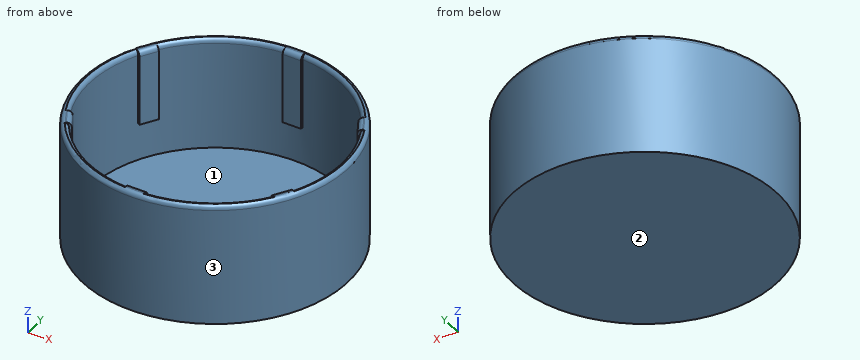
from build123d import *

# Parameters (mm, degrees)
F0_R         = 7.1
F1_DEPTH     = 0.5
F2_R         = 7.1
F2_R_2       = 6.7
F3_DEPTH     = 6
F4_W         = 1
F4_H         = 0.3
F5_DEPTH     = 4
F6_R         = 0.25
F7_T4_ANGLE  = 62.1313472273
F7_T10_ANGLE = 62.1313472273
F7_T16_ANGLE = 62.1313472273
F7_T22_ANGLE = 62.1313472273
F7_T28_ANGLE = 31.0651476548
F7_T33_ANGLE = 62.1313472273
F7_T39_ANGLE = 31.0651476548
F8_R         = 0.25


# Not quite as in the source:
# - a fillet or chamfer that OpenCascade refuses, or shapes differently, is made with other operations: its cross-section is extruded or revolved along the edge and cut away or added


with BuildPart() as f1:
    # F0 (on Top) → F1 (new body)
    with BuildSketch(Plane.XY):
        Circle(F0_R)
    extrude(amount=F1_DEPTH)

    # F2 (on face) → F3 (join)
    with BuildSketch(Plane.XY.offset(0.5)):
        Circle(F2_R)
        Circle(F2_R_2, mode=Mode.SUBTRACT)
    extrude(amount=F3_DEPTH)

    # F4 (on face) → F5 (join)
    with BuildSketch(Plane.XY.offset(6.5)):
        with Locations((0, 6.7)):
            Rectangle(F4_W, F4_H)
        Polygon((-5.9224663948, 2.8419872981), (-5.4224663948, 3.7080127019), (-5.6822740159, 3.8580127019), (-6.1822740159, 2.9919872981), align=None)
        Polygon((-5.4224663948, -3.7080127019), (-5.9224663948, -2.8419872981), (-6.1822740159, -2.9919872981), (-5.6822740159, -3.8580127019), align=None)
        with Locations((0, -6.7)):
            Rectangle(F4_W, F4_H)
        Polygon((5.9224663948, -2.8419872981), (5.4224663948, -3.7080127019), (5.6822740159, -3.8580127019), (6.1822740159, -2.9919872981), align=None)
        Polygon((5.4224663948, 3.7080127019), (5.9224663948, 2.8419872981), (6.1822740159, 2.9919872981), (5.6822740159, 3.8580127019), align=None)
    extrude(amount=-F5_DEPTH)

    # F6
    f6_edges = [f1.edges().sort_by_distance(p)[0] for p in [
        (-7.1, 0, 6.5),
    ]]
    fillet(f6_edges, radius=F6_R)

    # F7: fillet of radius 0.25 on 6 edges, made by hand


with BuildPart() as f7_tool2:
    # F7_s3 → F7_t4 (revolve)
    with BuildSketch(Plane(origin=(0, 0, 0), x_dir=(0, 0, 1), z_dir=(-0.4838067947, 0.8751748313, 0))):
        with BuildLine():
            ThreePointArc((6.5, -6.95), (6.4267766953, -6.7732233047), (6.25, -6.7))
            Line((6.25, -6.7), (6.5, -6.7))
            Line((6.5, -6.7), (6.5, -6.95))
        make_face()
    revolve(axis=Axis((0, 0, 6.5), (0, 0, 1)), revolution_arc=F7_T4_ANGLE)

    split(bisect_by=Plane.YZ.offset(-0.5), keep=Keep.BOTTOM)

    split(bisect_by=Plane(origin=(0.25, -0.4330127019, 0), x_dir=(0, 0, 1), z_dir=(0.5, -0.8660254038, 0)), keep=Keep.TOP)


with BuildPart() as f1_1:
    add(f1.part)

    # F7_t1: cut F7_tool2
    add(f7_tool2.part, mode=Mode.SUBTRACT)


with BuildPart() as f7_tool8:
    # F7_s9 → F7_t10 (revolve)
    with BuildSketch(Plane(origin=(0, 0, 0), x_dir=(0, 0, 1), z_dir=(0.5160202393, 0.8565763904, 0))):
        with BuildLine():
            ThreePointArc((6.5, -6.95), (6.4267766953, -6.7732233047), (6.25, -6.7))
            Line((6.25, -6.7), (6.5, -6.7))
            Line((6.5, -6.7), (6.5, -6.95))
        make_face()
    revolve(axis=Axis((0, 0, 6.5), (0, 0, 1)), revolution_arc=F7_T10_ANGLE)

    split(bisect_by=Plane(origin=(-0.25, 0.4330127019, 0), x_dir=(0, 0, 1), z_dir=(-0.5, 0.8660254038, 0)), keep=Keep.TOP)

    split(bisect_by=Plane(origin=(-0.25, -0.4330127019, 0), x_dir=(0, 0, 1), z_dir=(-0.5, -0.8660254038, 0)), keep=Keep.TOP)


with BuildPart() as f1_2:
    add(f1_1.part)

    # F7_t7: cut F7_tool8
    add(f7_tool8.part, mode=Mode.SUBTRACT)


with BuildPart() as f7_tool14:
    # F7_s15 → F7_t16 (revolve)
    with BuildSketch(Plane(origin=(0, 0, 0), x_dir=(0, 0, 1), z_dir=(0.999827034, -0.0185984409, 0))):
        with BuildLine():
            ThreePointArc((6.5, -6.95), (6.4267766953, -6.7732233047), (6.25, -6.7))
            Line((6.25, -6.7), (6.5, -6.7))
            Line((6.5, -6.7), (6.5, -6.95))
        make_face()
    revolve(axis=Axis((0, 0, 6.5), (0, 0, 1)), revolution_arc=F7_T16_ANGLE)

    split(bisect_by=Plane(origin=(0.25, 0.4330127019, 0), x_dir=(0, 0, 1), z_dir=(0.5, 0.8660254038, 0)), keep=Keep.TOP)

    split(bisect_by=Plane.YZ.offset(-0.5), keep=Keep.BOTTOM)


with BuildPart() as f1_3:
    add(f1_2.part)

    # F7_t13: cut F7_tool14
    add(f7_tool14.part, mode=Mode.SUBTRACT)


with BuildPart() as f7_tool20:
    # F7_s21 → F7_t22 (revolve)
    with BuildSketch(Plane(origin=(0, 0, 0), x_dir=(0, 0, 1), z_dir=(0.4838067947, -0.8751748313, 0))):
        with BuildLine():
            ThreePointArc((6.5, -6.95), (6.4267766953, -6.7732233047), (6.25, -6.7))
            Line((6.25, -6.7), (6.5, -6.7))
            Line((6.5, -6.7), (6.5, -6.95))
        make_face()
    revolve(axis=Axis((0, 0, 6.5), (0, 0, 1)), revolution_arc=F7_T22_ANGLE)

    split(bisect_by=Plane.YZ.offset(0.5), keep=Keep.TOP)

    split(bisect_by=Plane(origin=(-0.25, 0.4330127019, 0), x_dir=(0, 0, 1), z_dir=(-0.5, 0.8660254038, 0)), keep=Keep.TOP)


with BuildPart() as f1_4:
    add(f1_3.part)

    # F7_t19: cut F7_tool20
    add(f7_tool20.part, mode=Mode.SUBTRACT)


with BuildPart() as f7_tool26:
    # F7_s27 → F7_t28 (revolve)
    with BuildSketch(Plane(origin=(0, 0, 0), x_dir=(0, 0, 1), z_dir=(-0.5160123762, -0.8565811273, 0))):
        with BuildLine():
            ThreePointArc((6.5, -6.95), (6.4267766953, -6.7732233047), (6.25, -6.7))
            Line((6.25, -6.7), (6.5, -6.7))
            Line((6.5, -6.7), (6.5, -6.95))
        make_face()
    revolve(axis=Axis((0, 0, 6.5), (0, 0, 1)), revolution_arc=F7_T28_ANGLE)

    split(bisect_by=Plane(origin=(0.25, 0.4330127019, 0), x_dir=(0, 0, 1), z_dir=(0.5, 0.8660254038, 0)), keep=Keep.TOP)


with BuildPart() as f1_5:
    add(f1_4.part)

    # F7_t25: cut F7_tool26
    add(f7_tool26.part, mode=Mode.SUBTRACT)


with BuildPart() as f7_tool31:
    # F7_s32 → F7_t33 (revolve)
    with BuildSketch(Plane(origin=(0, 0, 0), x_dir=(0, 0, 1), z_dir=(-0.999827034, 0.0185984409, 0))):
        with BuildLine():
            ThreePointArc((6.5, -6.95), (6.4267766953, -6.7732233047), (6.25, -6.7))
            Line((6.25, -6.7), (6.5, -6.7))
            Line((6.5, -6.7), (6.5, -6.95))
        make_face()
    revolve(axis=Axis((0, 0, 6.5), (0, 0, 1)), revolution_arc=F7_T33_ANGLE)

    split(bisect_by=Plane(origin=(-0.25, -0.4330127019, 0), x_dir=(0, 0, 1), z_dir=(-0.5, -0.8660254038, 0)), keep=Keep.TOP)

    split(bisect_by=Plane.YZ.offset(0.5), keep=Keep.TOP)


with BuildPart() as f1_6:
    add(f1_5.part)

    # F7_t30: cut F7_tool31
    add(f7_tool31.part, mode=Mode.SUBTRACT)


with BuildPart() as f7_tool37:
    # F7_s38 → F7_t39 (revolve)
    with BuildSketch(Plane.XZ):
        with BuildLine():
            ThreePointArc((6.95, 6.5), (6.7732233047, 6.4267766953), (6.7, 6.25))
            Line((6.7, 6.25), (6.7, 6.5))
            Line((6.7, 6.5), (6.95, 6.5))
        make_face()
    revolve(axis=Axis((0, 0, 6.5), (0, 0, 1)), revolution_arc=F7_T39_ANGLE)

    split(bisect_by=Plane(origin=(0.25, -0.4330127019, 0), x_dir=(0, 0, 1), z_dir=(0.5, -0.8660254038, 0)), keep=Keep.TOP)


with BuildPart() as f1_7:
    add(f1_6.part)

    # F7_t36: cut F7_tool37
    add(f7_tool37.part, mode=Mode.SUBTRACT)

    # F8
    f8_edges = [f1_7.edges().sort_by_distance(p)[0] for p in [
        (-5.672466, 3.275, 6.5),
        (0, 6.55, 6.5),
        (5.672466, 3.275, 6.5),
        (5.672466, -3.275, 6.5),
        (0, -6.55, 6.5),
        (-5.672466, -3.275, 6.5),
    ]]
    fillet(f8_edges, radius=F8_R)


solid = f1_7.part
The listing builds one solid part. Answer for the finished solid, in the listing's coordinates (mm). Face numbers are marked on the shaded views. Give positions to 0.01 mm unless a question says otherwise; leave off trailing zeros. Write each loop counter-clockwise with the first axis right and the second up, starting at its lowest first coordinate (ties: lowest second). Pieces come first, ordered by that corner, then holes.
Item 1: Section A-A, the plane x = 0 is taken. Write down the section's boundary in (y, z), plus the area to 3 significant figures.
Item 2: Find the intervals of material crossed by line 1 along Y through (x, z) = (0, 5.05); line 2 along Y through (x, z) = (0, 1.95); line 3 along X through (y, z) = (-6, 5), in increasing order.
Item 3: Flat-ended cylindrical pins translate along their axes: P1, Ø0.5, axis at x = 5.5, y = 3.5, coming from the -Z side; P2, Ø2, axis at y = 2.5, z = 5.5, coming from the +X side; P3, Ø1, axis at x = 2.5, z = 3, coming from the -Y side; P4, Ø3, axis at y = 5, z = 5, coming from the +X side. Find the tip coordinate at first contact, or state that the pin passes through.
Item 4: Determine the mould class of the marked faces 1, 2 and 3 for opening direction Y: released by +Y, released by -Y, zero draft, split by the parting line, or undercut.
Item 5: Section B-B, the plane z = 5.75 is taken. Write down the section's boundary in (x, y).
Item 6: Section C-C, the plane z = 1.75 is taken. Write down the section's boundary in (x, y), plus the area to 3 significant figures.
Completed:
1. outline: (-7.1, 0) - (7.1, 0) - (7.1, 6.25) arc R0.25 ccw to (6.85, 6.5) - (6.8, 6.5) arc R0.25 ccw to (6.55, 6.25) - (6.55, 2.5) - (6.7, 2.5) - (6.7, 0.5) - (-6.7, 0.5) - (-6.7, 2.5) - (-6.55, 2.5) - (-6.55, 6.25) arc R0.25 ccw to (-6.8, 6.5) - (-6.85, 6.5) arc R0.25 ccw to (-7.1, 6.25) - close
1. area: 13.0 mm2
2. line 1: y = -7.1 to -6.55, 6.55 to 7.1
2. line 2: y = -7.1 to -6.7, 6.7 to 7.1
2. line 3: x = -3.8 to -2.98, 2.98 to 3.8
3. P1: stops at z = 0
3. P2: stops at x = 6.94
3. P3: stops at y = -6.81
3. P4: stops at x = 6.18
4. face 1: undercut
4. face 2: zero draft
4. face 3: split by the parting line
5. outline: circle Ø14.2 at (0, 0); hole (-6.04, -2.91) - (-5.92, -2.84) - (-5.42, -3.71) - (-5.54, -3.77) arc R6.7 ccw to (-0.5, -6.68) - (-0.5, -6.55) - (0.5, -6.55) - (0.5, -6.68) arc R6.7 ccw to (5.54, -3.77) - (5.42, -3.71) - (5.92, -2.84) - (6.04, -2.91) arc R6.7 ccw to (6.04, 2.91) - (5.92, 2.84) - (5.42, 3.71) - (5.54, 3.77) arc R6.7 ccw to (0.5, 6.68) - (0.5, 6.55) - (-0.5, 6.55) - (-0.5, 6.68) arc R6.7 ccw to (-5.54, 3.77) - (-5.42, 3.71) - (-5.92, 2.84) - (-6.04, 2.91) arc R6.7 ccw to start
6. outline: circle Ø14.2 at (0, 0); hole circle Ø13.4 at (0, 0)
6. area: 17.3 mm2
